```python
from build123d import *

# Parameters (mm, degrees)
F1_DEPTH = 2
F2_R     = 4.1
F2_R_2   = 1.5
F3_DEPTH = 8
F5_DEPTH = 12


with BuildPart() as f1:
    # F0 (on Top) → F1 (new body)
    with BuildSketch(Plane.XY):
        with BuildLine():
            ThreePointArc((-16.1402020254, 4.1), (-20.1, 5.7), (-24.0597979746, 4.1))
            Line((-24.0597979746, 4.1), (-16.1402020254, 4.1))
        make_face()
        with BuildLine():
            Line((-16.1402020254, 4.1), (-24.0597979746, 4.1))
            ThreePointArc((-24.0597979746, 4.1), (-24.1051466384, 4.0557120713), (-24.15, 4.0109225871))
            ThreePointArc((-24.15, 4.0109225871), (-29.1, 0), (-24.15, -4.0109225871))
            ThreePointArc((-24.15, -4.0109225871), (-24.1051466384, -4.0557120713), (-24.0597979746, -4.1))
            Line((-24.0597979746, -4.1), (-16.1402020254, -4.1))
            Line((-16.1402020254, -4.1), (21.6402020254, -4.1))
            ThreePointArc((21.6402020254, -4.1), (19.9, 0), (21.6402020254, 4.1))
            Line((21.6402020254, 4.1), (-16.1402020254, 4.1))
        make_face()
        with BuildLine():
            Line((-16.1402020254, -4.1), (-24.0597979746, -4.1))
            ThreePointArc((-24.0597979746, -4.1), (-20.1, -5.7), (-16.1402020254, -4.1))
        make_face()
    extrude(amount=F1_DEPTH)

    # F2 (on face) → F3 (join)
    with BuildSketch(Plane.XY.offset(2)):
        with Locations((-25, 0)):
            Circle(F2_R)
        with Locations((-25, 0)):
            Circle(F2_R_2, mode=Mode.SUBTRACT)
    extrude(amount=F3_DEPTH)

    # F4 (on face) → F5 (join)
    with BuildSketch(Plane(origin=(0, 0, 0), x_dir=(1, 0, 0), z_dir=(0, 0, -1))):
        with BuildLine():
            Line((-23.8593048022, -1.7426615038), (-22.7605585052, -2.7))
            Line((-22.7605585052, -2.7), (-1.5, -2.7))
            Line((-1.5, -2.7), (-1.5, 2.3))
            Line((-1.5, 2.3), (-17.5988609143, 2.3))
            ThreePointArc((-17.5988609143, 2.3), (-17.986159249, 2.116227766), (-18.0887588629, 1.7))
            ThreePointArc((-18.0887588629, 1.7), (-19.4175132364, -1.1369373376), (-22.5168783934, -0.6811553006))
            Line((-22.5168783934, -0.6811553006), (-22.6406951978, -0.5573384962))
            ThreePointArc((-22.6406951978, -0.5573384962), (-23.8426615038, -0.5406951978), (-23.8593048022, -1.7426615038))
        make_face()
        with BuildLine():
            ThreePointArc((-15.5, -1.45), (-16.2071067812, -1.1571067812), (-16.5, -0.45))
            Line((-16.5, -0.45), (-16.5, -0.2))
            ThreePointArc((-16.5, -0.2), (-16.2071067812, 0.5071067812), (-15.5, 0.8))
            Line((-15.5, 0.8), (-10.75, 0.8))
            ThreePointArc((-10.75, 0.8), (-10.0428932188, 0.5071067812), (-9.75, -0.2))
            Line((-9.75, -0.2), (-9.75, -0.45))
            ThreePointArc((-9.75, -0.45), (-10.0428932188, -1.1571067812), (-10.75, -1.45))
            Line((-10.75, -1.45), (-15.5, -1.45))
        make_face(mode=Mode.SUBTRACT)
        with BuildLine():
            Line((-2.75, -0.2), (-2.75, -0.45))
            ThreePointArc((-2.75, -0.45), (-3.0428932188, -1.1571067812), (-3.75, -1.45))
            Line((-3.75, -1.45), (-7.5, -1.45))
            ThreePointArc((-7.5, -1.45), (-8.2071067812, -1.1571067812), (-8.5, -0.45))
            Line((-8.5, -0.45), (-8.5, -0.2))
            ThreePointArc((-8.5, -0.2), (-8.2071067812, 0.5071067812), (-7.5, 0.8))
            Line((-7.5, 0.8), (-3.75, 0.8))
            ThreePointArc((-3.75, 0.8), (-3.0428932188, 0.5071067812), (-2.75, -0.2))
        make_face(mode=Mode.SUBTRACT)
        with BuildLine():
            Line((0, 2.3), (0, -2.7))
            Line((0, -2.7), (23.7999915966, -2.72))
            Line((23.7999915966, -2.72), (23.7999915966, -1.47))
            ThreePointArc((23.7999915966, -1.47), (22.2959243854, 0.1440913013), (21.75, 2.281724448))
            Line((21.75, 2.281724448), (11.7499999993, 2.2901270007))
            Line((11.7499999993, 2.2901270007), (1.25, 2.2989496809))
            Line((1.25, 2.2989496809), (0, 2.3))
        make_face()
        with BuildLine():
            ThreePointArc((2.25, -1.47), (1.5428932188, -1.1771067812), (1.25, -0.47))
            Line((1.25, -0.47), (1.25, -0.2))
            ThreePointArc((1.25, -0.2), (1.5428932188, 0.5071067812), (2.25, 0.8))
            Line((2.25, 0.8), (9.5, 0.8))
            ThreePointArc((9.5, 0.8), (10.2071067812, 0.5071067812), (10.5, -0.2))
            Line((10.5, -0.2), (10.5, -0.47))
            ThreePointArc((10.5, -0.47), (10.2071067812, -1.1771067812), (9.5, -1.47))
            Line((9.5, -1.47), (2.25, -1.47))
        make_face(mode=Mode.SUBTRACT)
        with BuildLine():
            ThreePointArc((12.75, -1.47), (12.0428932188, -1.1771067812), (11.75, -0.47))
            Line((11.75, -0.47), (11.75, -0.2))
            ThreePointArc((11.75, -0.2), (12.0428932188, 0.5071067812), (12.75, 0.8))
            Line((12.75, 0.8), (19.5, 0.8))
            ThreePointArc((19.5, 0.8), (20.2071067812, 0.5071067812), (20.5, -0.2))
            Line((20.5, -0.2), (20.5, -0.47))
            ThreePointArc((20.5, -0.47), (20.2071067812, -1.1771067812), (19.5, -1.47))
            Line((19.5, -1.47), (12.75, -1.47))
        make_face(mode=Mode.SUBTRACT)
    extrude(amount=F5_DEPTH)


solid = f1.part
```
Input: part model. Units: mm. Frame: model coordinates. A direction names the side the tool comes from. Round coordinates to 2 decimals unless told otherwise and drop trailing zeros. Write each loop counter-clockwise with the first axis right and the second up, starting at its lowest first coordinate (ties: lowest second). Pieces come first, ordered by that corner, then holes. Notation, with made-up numbers: (44, 33.25) -> (98, 33.25) arc R21 cw to (98, 41.25) -> close; hole circle Ø3 at (43.25, 20.5). An arc over 180 degrees is marked (long way). Answer as CSV lines item,"result".
1. Contact query for flat-ended pins moving along their axis: P1, Ø3, axis at x = -22.5, z = -2, coming from the -Y side; P2, Ø2.5, axis at y = 0, z = -6, coming from the -X side; P3, Ø6, axis at x = -10, z = -9, coming from the -Y side. Output: stop coordinate, or through.
Geometry says:
P1,"stops at y = 0.3"
P2,"stops at x = -24.1"
P3,"stops at y = -2.3"
2. Reachability of faces 1 (the flat face through (-25, 0, 2)), 2 (the flat face through (-13, 0, 0)), 3 (the cylindrical face through (19.9, -0.1, 1)) from +Z, -Z, +X, -X, +Y, -Y: full face, straight path, thin tool, end or side. Return the list, or none.
Geometry says:
face 1,"+Z"
face 2,"-Z"
face 3,"+Z, +X"
3. Section B-B (z = 3.5). Return the cut outline in (x, y).
Geometry says:
outline,"circle Ø8.2 at (-25, 0); hole circle Ø3 at (-25, 0)"
4. Section C-C (y = -3). Return the cut outline in (x, z).
Geometry says:
outline,"(-27.79, 0) -> (20.75, 0) -> (20.75, 2) -> (-22.21, 2) -> (-22.21, 10) -> (-27.79, 10) -> close"
5. Ray query, L1, parallel to Y at x = -25, z = 8; L2, parallel to Y at x = 15, z = -8; L3, parallel to Z at x = -25.5, y = -3.25. Return the intervals inside material, ascending. Write a range as [from, to].
Geometry says:
L1,"y = [-4.1, -1.5], [1.5, 4.1]"
L2,"y = [-2.29, -0.8], [1.47, 2.71]"
L3,"z = [0, 10]"
6. Section A-A (x = -25). Return the cut outline in (y, z), plus the area to 3 significant figures.
Geometry says:
outline,"(-4.1, 0) -> (4.1, 0) -> (4.1, 10) -> (1.5, 10) -> (1.5, 2) -> (-1.5, 2) -> (-1.5, 10) -> (-4.1, 10) -> close"
area,"58.0 mm^2"
7. Section D-D (z = -2). Give the number of separate pieces and of enclosed holes in the cut face, plus the area to 3 significant figures.
Geometry says:
separate pieces,"2"
enclosed holes,"4"
area,"141 mm^2"
